Source: CAD feature listing. Evaluate the final solid. Frame: model axes, mm. A direction names the side the tool comes from. Give positions to 0.01 mm unless a question says otherwise; leave off trailing zeros. Loops run counter-clockwise (first coordinate to the right, second up) from the corner with the lowest first, then second, coordinate; pieces in that order, holes last. Notation, with made-up numbers: (39.5, 40.25) -> (85.5, 40.25) arc R21 cw to (85.5, 58.25) -> close; hole circle Ø8 at (-17.75, 77). An arc over 180 degrees is marked (long way). Answer as a JSON object with one key per item and string values. Group by question number.
from build123d import *

# Parameters (mm, degrees)
SKETCH1_W           = 34.036
SKETCH1_H           = 34.036
BOSS_EXTRUDE1_DEPTH = 203.2
SKETCH2_R           = 1
CUT_EXTRUDE1_DEPTH  = 38.1
FILLET1_R           = 2.54
SKETCH3_R           = 5.15
CUT_EXTRUDE2_DEPTH  = 190.5
SKETCH4_R           = 1.5875
CUT_EXTRUDE3_DEPTH  = 205.620293832


with BuildPart() as part:
    # Sketch1 → Boss-Extrude1 (new body)
    with BuildSketch(Plane(origin=(0, 0, 0), x_dir=(1, 0, 0), z_dir=(0, 1, 0))):
        Rectangle(SKETCH1_W, SKETCH1_H)
    extrude(amount=BOSS_EXTRUDE1_DEPTH)

    # Sketch2 → Cut-Extrude1 (cut)
    with BuildSketch(Plane(origin=(0, 203.2, 0), x_dir=(1, 0, 0), z_dir=(0, 1, 0))):
        with Locations(Location((0, 8, 0), (0, 0, 270))):
            Circle(SKETCH2_R)
        with Locations(Location((0, -8, 0), (0, 0, 270))):
            Circle(SKETCH2_R)
        with Locations(Location((-8, 0, 0), (0, 0, 270))):
            Circle(SKETCH2_R)
        with Locations(Location((8, 0, 0), (0, 0, 270))):
            Circle(SKETCH2_R)
    extrude(amount=-CUT_EXTRUDE1_DEPTH, mode=Mode.SUBTRACT)

    # Fillet1
    fillet1_edges = [part.edges().sort_by_distance(p)[0] for p in [
        (-17.018, 101.6, -17.018),
        (17.018, 101.6, -17.018),
        (17.018, 101.6, 17.018),
        (-17.018, 101.6, 17.018),
    ]]
    fillet(fillet1_edges, radius=FILLET1_R)

    # Sketch3 → Cut-Extrude2 (cut)
    with BuildSketch(Plane(origin=(0, 203.2, 0), x_dir=(1, 0, 0), z_dir=(0, 1, 0))):
        with Locations(Location((0, 0, 0), (0, 0, 270))):
            Circle(SKETCH3_R)
    extrude(amount=-CUT_EXTRUDE2_DEPTH, mode=Mode.SUBTRACT)

    # Sketch4 → Cut-Extrude3 (cut, through all)
    with BuildSketch(Plane.XZ):
        with Locations(Location((0, 0, 0), (0, 0, 270))):
            Circle(SKETCH4_R)
    extrude(amount=-CUT_EXTRUDE3_DEPTH, mode=Mode.SUBTRACT)


solid = part.part
(1) Section query A-A on y = 170.5. Return the cut outline in (x, z).
(2) Material intervals for line 1 (X direction, y = 194, z = 0); line 2 (X direction, y = 2.5, z = 0); line 3 (Z direction, x = 3.5, y = 131), sorted ascending. Write a range as from..to.
(3) Access query for faces 5 (the face through (-2, 12.7, 0)), 6 (the face through (0, 0, -4)). Directions: +Z, -Z, +X, -X, +Y, -Y. A direction counts if a zero-diameter tool reaches every point of the face in a straight line with its end or side. Return the directions, or none.
(4) Section query B-B on y = 20. Return the cut outline in (x, z).
(5) Mould query, pull axis Z, two halves, no side actions, for faces 1 (the face through (0, 100, 17.018)), 2 (the face through (17.018, 100, 0)), 3 (the face through (0, 100, -17.018)), 4 (the face through (-5.028, 109.283, -1.116)). Classes: pulls with the +Z half, pulls with the -Z half, needs draft (parallel to the pull), parting line crosses it, or undercut.
(6) First-contact query: pin 1 (9.5 mm diameter, centred on x = 0, z = 0, fed in from +Y). Flat tip, straight axial feed; report the tip coordinate or a pass-through.
Result:
{
 "1": {"outline": "(-17.02, -14.48) arc R2.54 ccw to (-14.48, -17.02) -> (14.48, -17.02) arc R2.54 ccw to (17.02, -14.48) -> (17.02, 14.48) arc R2.54 ccw to (14.48, 17.02) -> (-14.48, 17.02) arc R2.54 ccw to (-17.02, 14.48) -> close; hole circle Ø2 at (-8, 0); hole circle Ø10.3 at (0, 0); hole circle Ø2 at (0, -8); hole circle Ø2 at (0, 8); hole circle Ø2 at (8, 0)"},
 "2": {"line 1": "-17.02..-9, -7..-5.15, 5.15..7, 9..17.02", "line 2": "-17.02..-1.59, 1.59..17.02", "line 3": "-17.02..-3.78, 3.78..17.02"},
 "3": {"face 5": "+Y", "face 6": "+Z, -Z, +X, -X, -Y"},
 "4": {"outline": "(-17.02, -14.48) arc R2.54 ccw to (-14.48, -17.02) -> (14.48, -17.02) arc R2.54 ccw to (17.02, -14.48) -> (17.02, 14.48) arc R2.54 ccw to (14.48, 17.02) -> (-14.48, 17.02) arc R2.54 ccw to (-17.02, 14.48) -> close; hole circle Ø10.3 at (0, 0)"},
 "5": {"face 1": "pulls with the +Z half", "face 2": "needs draft", "face 3": "pulls with the -Z half", "face 4": "undercut"},
 "6": {"pin 1": "y = 12.7"}
}
